Read the model definition and answer for the solid it produces. Units are mm, in the model's axes. A direction names the side the tool comes from. Round coordinates to 2 decimals unless told otherwise and drop trailing zeros. Write each loop counter-clockwise with the first axis right and the second up, starting at its lowest first coordinate (ties: lowest second). Pieces come first, ordered by that corner, then holes. Notation, with made-up numbers: (34, 45.5) -> (85, 45.5) arc R25 ccw to (85, 60.5) -> close; hole circle Ø10 at (-32.5, 45.25). An arc over 180 degrees is marked (long way). Return JSON: item names as keys, results as strings. Group by question number.
(1) The mould has two halves that part along Y. Classify faces 3 (the flat face through (7.03, 7.11, -64.19)), 4 (the cylindrical face through (6.271, 6.528, -3.612)), 5 (the flat face through (5, 5, -130.2)): released by +Y, released by -Y, zero draft, split by the parting line, or undercut.
(2) Given pin 1 (2 mm diameter, centred on y = 7.5, z = -33.5, fed in from -X); pin 2 (8 mm diameter, centred on x = -2.5, y = -3, fed in from +Z), each flat-ended and moving along its own axis, determine where each tip first touches the part or whether it passes through.
(3) A cutting plane is placed at C-C on z = -89.5. Give the vertices of the cut face in (x, y), then the cut area to 3 significant figures.
(4) For faces 1 (the flat face through (7.11, -7.03, -64.19)), 2 (the flat face through (6, -3, -128.2)), determine the directions among +Z, -Z, +X, -X, +Y, -Y from which every point of the face is accessible in a straight line to the end or side of a thin tool.
(5) Straight lines are drawn through the part: line 1 (Y direction, x = 0, z = -55); line 2 (Z direction, x = 6.75, y = 1.25); line 3 (Y direction, x = 0, z = -129.8). For each, find the intervals that lie inside material, in ascending order.
(6) A cutting plane is placed at A-A on y = 0. Give the vertices of the cut face in (x, z), then the cut area to 3 significant figures.
```python
from build123d import *

# Parameters (mm, degrees)
SKETCH1_R           = 8.25
BOSS_EXTRUDE1_DEPTH = 128.2
BOSS_EXTRUDE2_DEPTH = 2
SKETCH6_R           = 1.4
CUT_EXTRUDE2_DEPTH  = 133.419344178
CIRPATTERN1_COUNT   = 2
CIRPATTERN1_ANGLE   = 270
SKETCH7_R           = 6.269832862
CUT_EXTRUDE3_DEPTH  = 131.965797161


with BuildPart() as part:
    # Sketch1 → Boss-Extrude1 (new body)
    with BuildSketch(Plane.XY):
        Polygon((10, 4.142135624), (4.142135624, 10), (-4.142135624, 10), (-10, 4.142135624), (-10, -4.142135624), (-4.142135624, -10), (4.142135624, -10), (10, -4.142135624), align=None)
        Circle(SKETCH1_R, mode=Mode.SUBTRACT)
    extrude(amount=-BOSS_EXTRUDE1_DEPTH)

    # Sketch2 → Boss-Extrude2 (add)
    with BuildSketch(Plane(origin=(0, 0, -128.2), x_dir=(-1, 0, 0), z_dir=(0, 0, -1))):
        Polygon((-10, 4.142135624), (-10, -4.142135624), (-4.142135624, -10), (4.142135624, -10), (10, -4.142135624), (10, 4.142135624), (4.142135624, 10), (-4.142135624, 10), align=None)
    extrude(amount=BOSS_EXTRUDE2_DEPTH)

    # Sketch6 → Cut-Extrude2 (cut, through all)
    with BuildSketch(Plane(origin=(-7.071067812, 7.071067812, 0), x_dir=(0, 0, 1), z_dir=(-0.7071067811865476, 0.7071067811865476, 0))):
        with Locations(Location((-13, 0, 0), (0, 0, 270))):
            Circle(SKETCH6_R)
        with Locations(Location((-5, 0, 0), (0, 0, 270))):
            Circle(SKETCH6_R)
        with Locations(Location((-115.2, 0, 0), (0, 0, 270))):
            Circle(SKETCH6_R)
        with Locations(Location((-123.2, 0, 0), (0, 0, 270))):
            Circle(SKETCH6_R)
    cut_extrude2 = extrude(amount=-CUT_EXTRUDE2_DEPTH, mode=Mode.SUBTRACT)

    # CirPattern1: Cut-Extrude2 ×2 about axis
    cirpattern1_axis = Axis((0, 0, 6.85), (0, 0, -1))
    for i in range(1, CIRPATTERN1_COUNT):
        add(cut_extrude2.rotate(cirpattern1_axis, i * CIRPATTERN1_ANGLE / (CIRPATTERN1_COUNT - 1)), mode=Mode.SUBTRACT)

    # Sketch7 → Cut-Extrude3 (cut, through all)
    with BuildSketch(Plane(origin=(0, 0, -130.2), x_dir=(-1, 0, 0), z_dir=(0, 0, -1))):
        Circle(SKETCH7_R)
    extrude(amount=-CUT_EXTRUDE3_DEPTH, mode=Mode.SUBTRACT)


solid = part.part
```
Checks:
{
 "1": {"face 3": "released by +Y", "face 4": "undercut", "face 5": "zero draft"},
 "2": {"pin 1": "stops at x = -7.64", "pin 2": "stops at z = -128.2"},
 "3": {"outline": "(-10, -4.14) -> (-4.14, -10) -> (4.14, -10) -> (10, -4.14) -> (10, 4.14) -> (4.14, 10) -> (-4.14, 10) -> (-10, 4.14) -> close; hole circle Ø16.5 at (0, 0)", "area": "118 mm^2"},
 "4": {"face 1": "+Z, -Z, +X, -Y", "face 2": "+Z"},
 "5": {"line 1": "y = -10 to -8.25, 8.25 to 10", "line 2": "z = -130.2 to -128.2", "line 3": "y = -10 to -6.27, 6.27 to 10"},
 "6": {"outline": "(-10, -130.2) -> (-6.27, -130.2) -> (-6.27, -128.2) -> (-8.25, -128.2) -> (-8.25, 0) -> (-10, 0) -> close; (6.27, -130.2) -> (10, -130.2) -> (10, 0) -> (8.25, 0) -> (8.25, -128.2) -> (6.27, -128.2) -> close", "area": "464 mm^2"}
}
